Autodesk Inventor part; units mm, degrees
ref_plane "YZ Plane" through (0, 0, 0) normal (1, 0, 0) x (0, 1, 0)
ref_plane "XZ Plane" through (0, 0, 0) normal (0, 1, 0) x (-1, 0, 0)
ref_plane "XY Plane" through (0, 0, 0) normal (0, 0, 1) x (1, 0, 0)
sketch "Sketch1" plane through (0, 0, 0) normal (0, 0, 1) x (1, 0, 0)
  line L0 (0, 0) -> (25.4, 0)
  line L1 (25.4, 0) -> (25.4, 25.4)
  line L2 (25.4, 25.4) -> (0, 25.4)
  line L3 (0, 25.4) -> (0, 0)
  line L4 (1.5875, 23.8125) -> (23.8125, 23.8125)
  line L5 (23.8125, 23.8125) -> (23.8125, 1.5875)
  line L6 (23.8125, 1.5875) -> (1.5875, 1.5875)
  line L7 (1.5875, 1.5875) -> (1.5875, 23.8125)
  dimension "d0" = 25.4
  dimension "d1" = 25.4
  dimension "d2" = 1.5875
extrude "Extrusion1" add sketch "Sketch1" along normal blind 317.5
sketch "Sketch2" plane through (25.4, 0, 0) normal (1, 0, 0) x (0, 0, -1)
  line L0 (0, 0) -> (0, 25.4)
  line L1 (0, 25.4) -> (0, 0)
  line L2 (0, 25.4) -> (-317.5, 25.4)
  line L3 (-317.5, 25.4) -> (-298.45, 0)
  line L4 (-317.5, 23.8125) -> (-317.5, 1.5875)
  line L5 (-298.45, 0) -> (-317.5, 0)
  line L6 (-317.5, 0) -> (-317.5, 25.4)
  line L7 (-317.5, 25.4) -> (-317.5, 0)
  line L8 (0, 25.4) -> (-20.32, 10.16)
  line L9 (-20.32, 10.16) -> (-12.7, 0)
  line L10 (0, 0) -> (-317.5, 0)
  line L11 (-12.7, 0) -> (0, 0)
  dimension "d6" = 36.87
  dimension "d9" = 53.13
  dimension "d10" = 25.4
extrude "Extrusion3" cut sketch "Sketch2" against normal blind 25.4 contours L10 L9 L8 L0 | L3 L5 L6 L4
properties part number "angle support" material "Aluminum 6061"
Check sheet for the modelled part. Datum: model origin and axes. Units: mm. A direction names the side the tool comes from. Round coordinates to 2 decimals unless told otherwise and drop trailing zeros. Order: outer loops, then holes, each group sorted by start corner. A loop starts at its lowest first (then second) coordinate and runs counter-clockwise, first axis right, second up.
Q1. Cross-section at A-A, the plane x = 9. Enter the section's corners in (y, z), plus the area to 3 significant figures.
Filled sheet:
outline: (0, 12.7) - (1.59, 13.89) - (1.59, 299.64) - (0, 298.45) - close; (23.81, 2.12) - (25.4, 0) - (25.4, 317.5) - (23.81, 316.31) - close
area: 955 mm2
Q2. Cross-section at C-C, the plane z = 260.5. Enter the section's corners in (x, y), plus the area to 3 significant figures.
Filled sheet:
outline: (0, 0) - (25.4, 0) - (25.4, 25.4) - (0, 25.4) - close; hole (1.59, 1.59) - (23.81, 1.59) - (23.81, 23.81) - (1.59, 23.81) - close
area: 151 mm2
Q3. Draft check along Y on faces 4 (the face through (24.05, 12.76, 308.02)), 5 (the face through (25.4, 13, 157)), 6 (the face through (13, 1.588, 155)). Enter one of: pulls with the +Y half, pulls with the -Y half, needs draft (parallel to the pull), parting line crosses it, or undercut.
Filled sheet:
face 4: pulls with the -Y half
face 5: needs draft
face 6: undercut
Q4. Depth check by flat-ended pin: P1, Ø12, axis at x = 13, z = 58.5, coming from the -Y side. Enter the tip coordinate at first touch or a pass-through.
Filled sheet:
P1: stops at y = 0
Q5. Set-up check for faces 1 (the face through (12.759, 1.341, 13.706)), 2 (the face through (13, 23.812, 157)), 3 (the face through (13, 25.4, 157)): record each of +Z, -Z, +X, -X, +Y, -Y from which the full face is reachable in a straight line by a thin tool's end or side.
Filled sheet:
face 1: -Z, +X, -X
face 2: +Z, -Z
face 3: +Z, -Z, +X, -X, +Y
Q6. Cross-section at B-B, the plane y = 13.5. Enter the section's corners in (x, z) (1 decimal), plus the area to 3 significant figures.
Filled sheet:
outline: (0, 15.9) - (1.6, 15.9) - (1.6, 308.6) - (0, 308.6) - close; (23.8, 15.9) - (25.4, 15.9) - (25.4, 308.6) - (23.8, 308.6) - close
area: 929 mm2
Q7. Scan lines: L1, parallel to X at y = 16.75, z = 163; L2, parallel to Z at x = 24.25, y = 13.75. Record each from-to range of solid material in increasing order.
Filled sheet:
L1: x = 0 to 1.59, 23.81 to 25.4
L2: z = 15.53 to 308.76
